from build123d import *

# Parameters (mm, degrees)
PRIMARY_SKETCH_W      = 19.05
PRIMARY_SKETCH_H      = 4.7498
PRIMARY_REVOLVE_ANGLE = 180
EDGE_CHAMFER_SIZE     = 0.381


with BuildPart() as part:
    # Primary Sketch → Primary Revolve (revolve)
    with BuildSketch(Plane.XY):
        with Locations((9.525, 10.3251)):
            Rectangle(PRIMARY_SKETCH_W, PRIMARY_SKETCH_H)
    revolve(axis=Axis((0, 0, 0), (1, 0, 0)), revolution_arc=PRIMARY_REVOLVE_ANGLE)

    # Edge Chamfer
    edge_chamfer_edges = [part.edges().sort_by_distance(p)[0] for p in [
        (19.05, 0, 12.7),
        (0, 0, 12.7),
    ]]
    chamfer(edge_chamfer_edges, length=EDGE_CHAMFER_SIZE)


solid = part.part
Can you work these out from the model? Positions are in its coordinate system, mm. Round coordinates to 2 decimals unless told otherwise and drop trailing zeros. Write each loop counter-clockwise with the first axis right and the second up, starting at its lowest first coordinate (ties: lowest second). Pieces come first, ordered by that corner, then holes. Notation, with made-up numbers: (81.25, 70.25) - (114.25, 70.25) arc R11 ccw to (114.25, 86.25) - close; hole circle Ø2 at (10.5, 33.25). An arc over 180 degrees is marked (long way). Write each question's results on one line, items separated by ' | '. Start each with the question number.
1) We'd pull the mould along Y, two halves only. Please class faces 1 (the cylindrical face through (9.66, 0.17, 7.95)), 2 (the flat face through (9, -10, 0)), 3 (the cylindrical face through (9.653, 0.279, 12.697)): released by +Y, released by -Y, zero draft, split by the parting line, or undercut.
2) Suppose I cut it at A-A (y = 0). List the corners of the cut face in (x, z) for me.
3) Suppose I cut it at B-B (x = 8.5). List the corners of the cut face in (y, z) for me, and give its area (3 significant figures).
4) For pin 1 Ø1 at (x, y) = (15, 2) entering from -Z; pin 2 Ø4 at (x, y) = (8.5, 4.5) entering from +Z; pin 3 Ø1.5 at (x, y) = (2.5, -1) entering from -Z, each with a flat end and sliding along its axis, tell me the tip position at first contact or that it passes through.
5) Please list where these lines run through material, in increasing order: line 1 (Y direction, x = 14, z = 4.75); line 2 (Y direction, x = 12, z = 5.5); line 3 (Z direction, x = 2, y = 2).
Here are the results:
1) face 1: undercut | face 2: zero draft | face 3: split by the parting line
2) outline: (0, 7.95) - (19.05, 7.95) - (19.05, 12.32) - (18.67, 12.7) - (0.38, 12.7) - (0, 12.32) - close
3) outline: (-12.7, 0) - (-7.95, 0) arc R7.95 cw to (7.95, 0) - (12.7, 0) arc R12.7 ccw to start | area: 154 mm2
4) pin 1: stops at z = 7.55 | pin 2: stops at z = 12.45 | pin 3: stops at z = 7.76
5) line 1: y = -11.78 to -6.38, 6.38 to 11.78 | line 2: y = -11.45 to -5.74, 5.74 to 11.45 | line 3: z = 7.69 to 12.54
